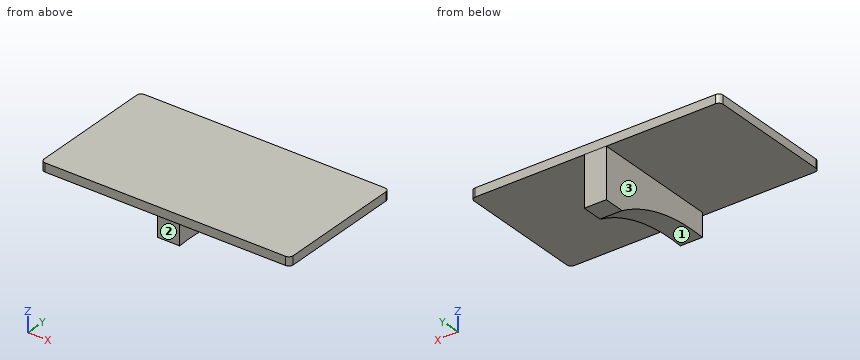
from build123d import *

# Parameters (mm, degrees)
F0_W     = 287.692204
F0_H     = 152.760788
F1_DEPTH = 10
F2_R     = 5.08
F4_DEPTH = 12.7


with BuildPart() as f1:
    # F0 (on Top) → F1 (new body)
    with BuildSketch(Plane.XY):
        Rectangle(F0_W, F0_H)
    extrude(amount=F1_DEPTH)

    # F2
    f2_edges = [f1.edges().sort_by_distance(p)[0] for p in [
        (143.846102, -76.380394, 5),
        (-143.846102, 76.380394, 5),
        (-143.846102, -76.380394, 5),
        (143.846102, 76.380394, 5),
    ]]
    fillet(f2_edges, radius=F2_R)

    # F3 (on Right) → F4 (join, symmetric)
    with BuildSketch(Plane.YZ):
        with BuildLine():
            Line((76.528475, 0), (0, 0))
            Line((0, 0), (-71.380883, 0))
            Line((-71.380883, 0), (-71.380883, -26.993327))
            ThreePointArc((-71.380883, -26.993327), (-7.032306, -32.181445), (52.20481, -57.845037))
            Line((52.20481, -57.845037), (76.528475, -57.845037))
            Line((76.528475, -57.845037), (76.528475, 0))
        make_face()
    extrude(amount=F4_DEPTH, both=True)


solid = f1.part
Read the model definition and answer for the solid it produces. Units are mm, in the model's axes. Face numbers are marked on the shaded views. Give positions to 0.01 mm unless a question says otherwise; leave off trailing zeros. Write each loop counter-clockwise with the first axis right and the second up, starting at its lowest first coordinate (ties: lowest second). Pieces come first, ordered by that corner, then holes. Notation, with made-up numbers: M -3,-26.75 L 51,-26.75 A22 cw 51,2.25 Z; hole C 38,82.5 d9. An arc over 180 degrees is marked long. One line per item, written item: value. Start each with the question number.
(1) Find section A-A (y = 59.5). Determine the outline of the cut face in (x, z), plus the area to 3 significant figures.
(2) Find section C-C (y = -64). Determine the outline of the cut face in (x, z).
(3) Flat-ended cylindrical pins translate along their axes: pin 1 Ø5 at (x, y) = (77, 35) entering from -Z; pin 2 Ø3 at (x, z) = (36, 5) entering from +Y; pin 3 Ø17.5 at (y, z) = (23, -26.5) entering from -X. Find the tip coordinate at first contact, or state that the pin passes through.
(4) Find section B-B (x = -6.5). Determine the outline of the cut face in (y, z), plus the area to 3 significant figures.
(5) Find section D-D (z = -35). Determine the outline of the cut face in (x, y), plus the area to 3 significant figures.
(6) Find the intervals of material crossed by line 1 (X direction, y = 11.5, z = -12); line 2 (Z direction, x = 116, y = -39); line 3 (Y direction, x = 0.5, z = -1.5), in increasing order.
(7) Determine the mould class of the marked faces 1, 2 and 3 for opening direction Y: pulls with the +Y half, pulls with the -Y half, needs draft (parallel to the pull), parting line crosses it, or undercut.
Results below:
1. outline: M -143.85,0 L -12.7,0 L -12.7,-57.85 L 12.7,-57.85 L 12.7,0 L 143.85,0 L 143.85,10 L -143.85,10 Z
1. area: 4,350 mm^2
2. outline: M -143.85,0 L -12.7,0 L -12.7,-26.51 L 12.7,-26.51 L 12.7,0 L 143.85,0 L 143.85,10 L -143.85,10 Z
3. pin 1: stops at z = 0
3. pin 2: stops at y = 76.38
3. pin 3: stops at x = -12.7
4. outline: M -76.38,0 L -71.38,0 L -71.38,-26.99 A197.48 cw 52.2,-57.85 L 76.53,-57.85 L 76.53,0 L 76.38,0 L 76.38,10 L -76.38,10 Z
4. area: 7,280 mm^2
5. outline: M -12.7,3.1 L 12.7,3.1 L 12.7,76.53 L -12.7,76.53 Z
5. area: 1,870 mm^2
6. line 1: x = -12.7 to 12.7
6. line 2: z = 0 to 10
6. line 3: y = -71.38 to 76.53
7. face 1: undercut
7. face 2: pulls with the -Y half
7. face 3: needs draft
